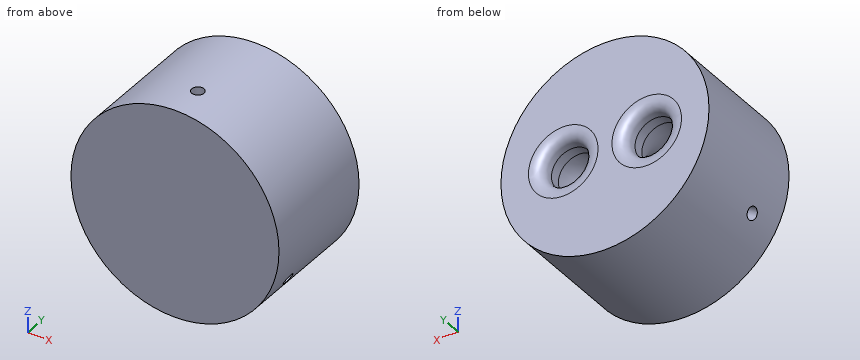
from build123d import *

# Parameters (mm, degrees)
SKETCH1_R           = 18.9865
BOSS_EXTRUDE1_DEPTH = 17.78
SKETCH2_R           = 3.81
SKETCH3_R           = 18.9865
SKETCH3_R_2         = 3.81
BOSS_EXTRUDE2_DEPTH = 4.445
FILLET1_SIZE        = 2.54
CIRPATTERN1_COUNT   = 3


with BuildPart() as part:
    # Sketch1 → Boss-Extrude1 (new body)
    with BuildSketch(Plane(origin=(0, 0, 0), x_dir=(1, 0, 0), z_dir=(0, 1, 0))):
        with Locations(Location((0, 0, 0), (0, 0, 270))):
            Circle(SKETCH1_R)
    extrude(amount=BOSS_EXTRUDE1_DEPTH)

    # Sketch2 → Cut-Revolve1 (revolve, cut)
    with BuildSketch(Plane(origin=(0, 17.78, 0), x_dir=(1, 0, 0), z_dir=(0, 1, 0)), mode=Mode.PRIVATE) as cut_revolve1_sk:
        with Locations((-7.62, 0)):
            Circle(SKETCH2_R)
    revolve(cut_revolve1_sk.sketch.rotate(Axis((0, 17.78, -18.9865), (0, 0, 1)), 90), axis=Axis((0, 17.78, -18.9865), (0, 0, 1)), mode=Mode.SUBTRACT)

    # Sketch3 → Boss-Extrude2 (add)
    with BuildSketch(Plane(origin=(0, 17.78, 0), x_dir=(1, 0, 0), z_dir=(0, 1, 0))):
        with Locations(Location((0, 0, 0), (0, 0, 270))):
            Circle(SKETCH3_R)
        with Locations((7.62, 0)):
            Circle(SKETCH3_R_2, mode=Mode.SUBTRACT)
        with Locations(Location((-7.62, 0, 0), (0, 0, 180))):
            Circle(SKETCH3_R_2, mode=Mode.SUBTRACT)
    extrude(amount=BOSS_EXTRUDE2_DEPTH)

    # Fillet1
    # a fillet whose section is not a circle: 2.54 mm, written as the material it takes off along each edge
    with BuildSketch(Plane(origin=(7.62, 22.225, 0), x_dir=(1, 0, 0), z_dir=(0, 0, 1))) as fillet1_piece_1:
        with BuildLine():
            add(Edge.make_bspline([(3.81 + FILLET1_SIZE, 0), (3.81 + FILLET1_SIZE * 0.831801948466, 0), (3.81 + FILLET1_SIZE * 0.663603896932, 0), (3.81 + FILLET1_SIZE * 0.292893218813, -FILLET1_SIZE * 0.0716919198361), (3.81 + FILLET1_SIZE * 0.0716919198361, -FILLET1_SIZE * 0.292893218813), (3.81, -FILLET1_SIZE * 0.663603896932), (3.81, -FILLET1_SIZE * 0.831801948466), (3.81, -FILLET1_SIZE)], knots=[0, 0, 0, 0, 0, 0, 0.5, 0.5, 1, 1, 1, 1, 1, 1], degree=5))
            Line((3.81, -FILLET1_SIZE), (3.81, 0))
            Line((3.81, 0), (3.81 + FILLET1_SIZE, 0))
        make_face()
    revolve(axis=Axis((7.62, 22.225, 0), (0, 1, 0)), mode=Mode.SUBTRACT)
    with BuildSketch(Plane(origin=(-7.62, 22.225, 0), x_dir=(-1, 0, 0), z_dir=(0, 0, -1))) as fillet1_piece_2:
        with BuildLine():
            add(Edge.make_bspline([(3.81 + FILLET1_SIZE, 0), (3.81 + FILLET1_SIZE * 0.831801948466, 0), (3.81 + FILLET1_SIZE * 0.663603896932, 0), (3.81 + FILLET1_SIZE * 0.292893218813, -FILLET1_SIZE * 0.0716919198361), (3.81 + FILLET1_SIZE * 0.0716919198361, -FILLET1_SIZE * 0.292893218813), (3.81, -FILLET1_SIZE * 0.663603896932), (3.81, -FILLET1_SIZE * 0.831801948466), (3.81, -FILLET1_SIZE)], knots=[0, 0, 0, 0, 0, 0, 0.5, 0.5, 1, 1, 1, 1, 1, 1], degree=5))
            Line((3.81, -FILLET1_SIZE), (3.81, 0))
            Line((3.81, 0), (3.81 + FILLET1_SIZE, 0))
        make_face()
    revolve(axis=Axis((-7.62, 22.225, 0), (0, 1, 0)), mode=Mode.SUBTRACT)

    # Sketch5 → Tap Drill for #4-40 Tap1 (revolve, cut)
    with BuildSketch(Plane(origin=(0, 6.35, 18.9865), x_dir=(0, -1, 0), z_dir=(1, 0, 0))):
        Polygon((0, 0), (0, 10.204152758), (1.1303, 9.525), (1.1303, 0), align=None)
    tap_drill_for_4_40_tap1 = revolve(axis=Axis((0, 6.35, 25.3365), (0, 0, -1)), mode=Mode.SUBTRACT)

    # CirPattern1: Tap Drill for #4-40 Tap1 ×3 about axis
    cirpattern1_axis = Axis((0, 0, 0), (0, -1, 0))
    for i in range(1, CIRPATTERN1_COUNT):
        add(tap_drill_for_4_40_tap1.rotate(cirpattern1_axis, i * 360 / CIRPATTERN1_COUNT), mode=Mode.SUBTRACT)


solid = part.part
Source: CAD feature listing. Evaluate the final solid. Frame: model axes, mm. Round coordinates to 2 decimals unless told otherwise and drop trailing zeros. Write each loop counter-clockwise with the first axis right and the second up, starting at its lowest first coordinate (ties: lowest second). Pieces come first, ordered by that corner, then holes. Notation, with made-up numbers: M 35,-22.75 L 64,-22.75 A33 cw 64,8.25 Z; hole C 67,68 d4. An arc over 180 degrees is marked long. One line per item, written item: value. Start each with the question number.
Item 1: Section query A-A (z = -13). Return the cut outline in (x, y) (3 decimals), plus the area to 3 significant figures.
Item 2: Section query B-B (y = 21.25). State how many separate pieces and enclosed holes the cut face has, plus the area to 3 significant figures.
Item 3: Pin query (flat end, axial travel): pin 1 (12 mm diameter, centred on x = -7.62, z = 0, fed in from +Y); pin 2 (5 mm diameter, centred on x = -9, y = 19.5, fed in from -Z); pin 3 (6 mm diameter, centred on y = 9.5, z = -2, fed in from +X). Return the tip coordinate at first contact, or that it passes through.
Item 4: Ray query, L1, parallel to X at y = 19.15, z = 0; L2, parallel to Y at x = 0, z = 14 (3 decimals); L3, parallel to Y at x = -6, z = 6. Return the intervals inside material, ascending. Write a range as from..to.
Result set:
1. outline: M -13.838,0 L 13.838,0 L 13.838,22.225 L -13.838,22.225 Z
1. area: 615 mm²
2. separate pieces: 1
2. enclosed holes: 2
2. area: 1,030 mm²
3. pin 1: stops at y = 22.22
3. pin 2: stops at z = -17.84
3. pin 3: stops at x = 18.99
4. L1: x = -18.99..-11.43, -3.81..3.81, 11.43..18.99
4. L2: y = 0..5.22, 7.48..22.225
4. L3: y = 0..22.22
